from build123d import *

# Parameters (mm, degrees)
F2_DEPTH = 6


with BuildPart() as f2:
    # F1 (on Front) → F2 (new body, symmetric)
    with BuildSketch(Plane.XZ):
        with BuildLine():
            Line((-1084.126008, -161.892822), (-1159.007441, -250))
            ThreePointArc((-1159.007441, -250), (23.455407, -358.460153), (1205.918255, -250))
            Line((1205.918255, -250), (1119.557507, -163.89909))
            ThreePointArc((1119.557507, -163.89909), (17.628749, -258.457501), (-1084.126008, -161.892822))
        make_face()
        Polygon((-1244.906732, 279.848588), (-1359.19107, 300), (-1159.007441, -250), (-1084.126008, -161.892822), align=None)
        Polygon((1119.557507, -163.89909), (1205.918255, -250), (1276.449047, 150), (1174.906386, 150), align=None)
    extrude(amount=F2_DEPTH, both=True)


solid = f2.part
CAD build for the part. Positions are in the model's coordinates, mm. Give positions to 0.01 mm unless a question says otherwise; leave off trailing zeros. Order: outer loops, then holes, each group sorted by start corner. A loop starts at its lowest first (then second) coordinate and runs counter-clockwise, first axis right, second up. Notation, with made-up numbers: (-31.5, 40) -> (-11.5, 40) arc R26 cw to (-11.5, 65) -> close; hole circle Ø1 at (35, -26). An arc over 180 degrees is marked (long way). Return JSON: item names as keys, results as strings.
Q1. Saw through at D-D (z = 235). Write the cut outline in (x, y), then the cut area to 3 significant figures.
Working result:
{"outline": "(-1335.53, -6) -> (-1228.58, -6) -> (-1228.58, 6) -> (-1335.53, 6) -> close", "area": "1,280 mm²"}
Q2. Saw through at C-C (x = 998). Write the cut outline in (y, z), then the cut area to 3 significant figures.
Working result:
{"outline": "(-6, -284.99) -> (6, -284.99) -> (6, -183.83) -> (-6, -183.83) -> close", "area": "1,210 mm²"}
Q3. Drill centre lines: line 1 (X direction, y = -0.5, z = 2); line 2 (X direction, y = 5.75, z = 136); line 3 (Z direction, x = 69, y = 0.5). Where is each one in solid material? Low to high.
Working result:
{"line 1": "-1250.73 to -1143.78, 1148.81 to 1250.35", "line 2": "-1299.5 to -1192.55, 1172.44 to 1273.98", "line 3": "-358.3 to -258.3"}
Q4. Mould opens along X. For faces 1 (the face through (6.81, -0.08, -358.44)), 2 (the face through (-1163.391, -0.084, 55.886)), 3 (the face through (-48, 6, -272)), 4 (the face through (1147.62, -0.08, -4.75)) say: pulls with the +X half, pulls with the -X half, needs draft (parallel to the pull), parting line crosses it, or undercut.
Working result:
{"face 1": "parting line crosses it", "face 2": "undercut", "face 3": "needs draft", "face 4": "undercut"}
Q5. Saw through at B-B (z = -119). Write the cut outline in (x, y), then the cut area to 3 significant figures.
Working result:
{"outline": "(-1206.69, -6) -> (-1099.74, -6) -> (-1099.74, 6) -> (-1206.69, 6) -> close; (1127.47, -6) -> (1229.02, -6) -> (1229.02, 6) -> (1127.47, 6) -> close", "area": "2,500 mm²"}
Q6. Saw through at A-A (y = 3). Write the cut outline in (x, z), then the cut area to 3 significant figures.
Working result:
{"outline": "(-1359.19, 300) -> (-1159.01, -250) arc R6500 ccw to (1205.92, -250) -> (1276.45, 150) -> (1174.91, 150) -> (1119.56, -163.9) arc R6400 cw to (-1084.13, -161.89) -> (-1244.91, 279.85) -> close", "area": "319,000 mm²"}
